Geometry check sheet. Reference: the model listing, model coordinates, mm. A direction names the side the tool comes from. Give positions to 0.01 mm unless a question says otherwise; leave off trailing zeros. Order: outer loops, then holes, each group sorted by start corner. A loop starts at its lowest first (then second) coordinate and runs counter-clockwise, first axis right, second up.
Autodesk Inventor part; units mm, degrees
ref_plane "Work Plane1" through (51.3469, 0, 0) normal (0, 0, -1) x (-1, 0, 0)
ref_plane "YZ Plane" through (0, 0, 0) normal (1, 0, 0) x (0, 1, 0)
ref_plane "XZ Plane" through (0, 0, 0) normal (0, 1, 0) x (-1, 0, 0)
sketch "Sketch1" plane through (0, 0, 0) normal (0, 0, 1) x (1, 0, 0)
  line L0 (-3.6884, 0) -> (19.2814, 0)
  line L1 (6.3771, 12) -> (4.5751, 15.8643)
  line L2 (6.3771, 12) -> (16, 12) construction
  line L3 (16, 12) -> (16, 0) construction
  arc A0 (4.5751, 15.8643) -> (0, 14.85) centre (2.4, 14.85) ccw
  line L4 (6.3771, 12) -> (6.3771, 0)
  line L5 (0, -3.5401) -> (0, 21.2403)
  point P0 (0, 0)
  dimension "d2" = 24
  dimension "d4" = 34.5
  dimension "d5" = 2.4
  dimension "d15" = 16
  dimension "d16" = 25
revolve "Ring" add sketch "Sketch1" angle 360 about axis through (-10, 0, 0) along (1, 0, 0)
sketch "Sketch2" plane through (0, 0, 0) normal (-1, 0, 0) x (0, 0, 1)
  circle A0 centre (0, 0) radius 4.9
  line L0 (-12, -6.9282) -> (-12, 6.9282)
  line L1 (-12, 6.9282) -> (0, 13.8564)
  line L2 (0, 13.8564) -> (12, 6.9282)
  line L3 (12, 6.9282) -> (12, -6.9282)
  line L4 (12, -6.9282) -> (0, -13.8564)
  line L5 (0, -13.8564) -> (-12, -6.9282)
  circle A1 centre (0, 0) radius 14.85
  dimension "d6" = 27.7128
extrude "Body" add sketch "Sketch2" against normal blind 16 contours A0 | L0 L1 L2 L3 L4 L5
sketch "Sketch3" plane through (0, 0, 0) normal (0, 0, 1) x (1, 0, 0)
  line L0 (5.5114, 13.8564) -> (16, 13.8564)
  line L1 (16, 6.9282) -> (16, 13.8564)
  line L2 (0, -14.85) -> (0, 14.85)
  line L3 (-3.2, 0) -> (19.2, 0)
  line L4 (14.9282, 13.8564) -> (16, 12)
  dimension "d10" = 30
  dimension "d11" = 24
revolve "Chamfer1" cut sketch "Sketch3" angle 360 about axis through (-10, 0, 0) along (1, 0, 0)
sketch "Sketch4" plane through (0, 0, 0) normal (-1, 0, 0) x (0, 0, 1)
  circle A0 centre (0, 0) radius 14.85
hole "Thread" at (0, 0, 0) direction (1, 0, 0) diameter 13.835 end through all
chamfer "Chamfer2" distance 1.0825 angle 30 1 edges at (0, 0, -6.9175) measured on face at (0, 12.0452, -1.4626)
ref_plane "Work Plane1" through (51.3469, 0, 0) normal (0, 0, -1) x (-1, 0, 0)
chamfer "Chamfer3" distance 1.0825 angle 45 1 edges at (16, 0, -6.9175)
equation "\"d6\" = 1.1547 * SW"
equation "\"d7\" = KOH"
equation "\"d12\" = -0.5 * GD1 + 0.5 * NND"
equation "\"d46\" = -0.5 * GD1 + 0.5 * NND"
equation "\"d51\" = -0.5 * GD1 + 0.5 * NND"
equation "\"d2\" = SW"
equation "\"d4\" = LADI"
equation "\"d5\" = PHH"
equation "\"d15\" = KOH"
equation "\"d16\" = KEWI"
equation "\"d10\" = ANG1"
equation "\"d11\" = SW0"
equation "\"ANG1\" = 30deg"
equation "\"KEWI\" = 25deg"
equation "\"NND\" = 16"
equation "\"LADI\" = 34.5"
equation "\"SW\" = 24"
equation "\"PHH\" = 2.4"
equation "\"KOH\" = NND"
equation "\"SW0\" = 24"
equation "\"d1\" = LADI"
equation "\"d3\" = PHH"
equation "\"GUL\" = 0.541266 * PTC"
equation "\"RR\" = PHH"
equation "\"THREADDIA\" = 16"
equation "\"TOA\" = 30deg"
equation "\"PTC\" = 2"
equation "\"GAL\" = 0.541266 * PTC"
equation "\"E0\" = 1.155 * SW"
properties part number "ISO 4161 - M16" material "Stainless Steel"
Item 1: Sectioned sample at A-A (x = 11.75). Enter the section's corners in (y, z) (1 decimal).
Reported:
outline: (-13.9, 0) - (-6.9, -12) - (6.9, -12) - (13.9, 0) - (6.9, 12) - (-6.9, 12) - close; hole circle Ø13.8 at (0, 0)
Item 2: Scan lines: L1, parallel to Y at x = 7.25, z = 0; L2, parallel to Z at x = 9, y = 0; L3, parallel to Y at x = 3.5, z = 6. Record each from-to range of solid material in increasing order.
Reported:
L1: y = -13.86 to -6.92, 6.92 to 13.86
L2: z = -12 to -6.92, 6.92 to 12
L3: y = -15.89 to -3.44, 3.44 to 15.89
Item 3: Gauge pin test, flat ends, axial feed: pin 1 (1 mm diameter, centred on y = 1.5, z = 5.5, fed in from +X); pin 2 (5 mm diameter, centred on x = 8, z = -5.5, fed in from +Y); pin 3 (4 mm diameter, centred on x = 2.5, y = 9.5, fed in from -Z); pin 4 (4 mm diameter, centred on y = -5.5, z = -1, fed in from -X). Record the tip position at first contact, or that the pin passes through.
Reported:
pin 1: passes through
pin 2: stops at y = 12.84
pin 3: stops at z = -15.53
pin 4: stops at x = 0.24
Item 4: Set-up check for faces 1 (the flat face through (10.682, -10.344, 6.084)), 2 (the flat face through (16, -8, 2)), 3 (the flat face through (10.682, 10.344, -6.084)), 4 (the flat face through (10.68, 10.44, 5.92)), 5 (the flat face through (10.68, -10.44, -5.92)): record each of +Z, -Z, +X, -X, +Y, -Y from which the full face is reachable in a straight line by a thin tool's end or side.
Reported:
face 1: +Z, +X, -Y
face 2: +Z, -Z, +X, +Y, -Y
face 3: -Z, +X, +Y
face 4: +Z, +X, +Y
face 5: -Z, +X, -Y
